from build123d import *

# Parameters (mm, degrees)
SKETCH2_R      = 7.9375
EXTRUDE1_DEPTH = 354.091885747
SKETCH3_R      = 186.436
SKETCH3_R_2    = 12.7
EXTRUDE2_DEPTH = 12.2936
SKETCH4_R      = 186.436
SKETCH4_R_2    = 12.7
EXTRUDE4_DEPTH = 26.9875
EXTRUDE5_START = -12.7
SKETCH5_R      = 186.436
EXTRUDE5_DEPTH = 12.7
EXTRUDE6_DEPTH = 351.045637854


with BuildPart() as part:
    # Sketch1 → Revolve1 (revolve)
    with BuildSketch(Plane(origin=(0, 0, 0), x_dir=(0, 0, -1), z_dir=(1, 0, 0)), mode=Mode.PRIVATE) as revolve1_sk:
        with BuildLine():
            Line((45.339, 0), (-45.339, 0))
            Line((-45.339, 0), (-45.339, 195.961))
            ThreePointArc((-45.339, 195.961), (0, 241.3), (45.339, 195.961))
            Line((45.339, 195.961), (45.339, 0))
        make_face()
    revolve(revolve1_sk.sketch.rotate(Axis((0, 0, 45.339), (0, 0, -1)), 90), axis=Axis((0, 0, 45.339), (0, 0, -1)))

    # Sketch2 → Extrude1 (cut, through all)
    with BuildSketch(Plane.XY.offset(45.339)):
        Circle(SKETCH2_R)
    extrude(amount=-EXTRUDE1_DEPTH, mode=Mode.SUBTRACT)

    # Sketch3 → Extrude2 (cut)
    with BuildSketch(Plane(origin=(0, 0, -45.339), x_dir=(-1, 0, 0), z_dir=(0, 0, -1))):
        Circle(SKETCH3_R)
        Circle(SKETCH3_R_2, mode=Mode.SUBTRACT)
    extrude(amount=-EXTRUDE2_DEPTH, mode=Mode.SUBTRACT)

    # Sketch4 → Extrude4 (cut)
    with BuildSketch(Plane(origin=(0, 0, -33.0454), x_dir=(-1, 0, 0), z_dir=(0, 0, -1))):
        Circle(SKETCH4_R)
        Circle(SKETCH4_R_2, mode=Mode.SUBTRACT)
    extrude(amount=-EXTRUDE4_DEPTH, mode=Mode.SUBTRACT)

    # Sketch5 → Extrude5 (cut)
    with BuildSketch(Plane.XY.offset(45.339).offset(EXTRUDE5_START)):
        with Locations(Location((0, 0, 0), (0, 0, 180))):
            Circle(SKETCH5_R)
    extrude(amount=EXTRUDE5_DEPTH, mode=Mode.SUBTRACT)

    # Sketch6 → Extrude6 (cut, through all)
    with BuildSketch(Plane.XY.offset(32.639)):
        with BuildLine():
            Line((150.489255243, 72.265671034), (80.015659908, 49.367411845))
            ThreePointArc((80.015659908, 49.367411845), (65.746331533, 21.36227807), (93.751465308, 7.092949695))
            Line((93.751465308, 7.092949695), (164.225060643, 29.991208884))
            ThreePointArc((164.225060643, 29.991208884), (158.770455984, 51.587648329), (150.489255243, 72.265671034))
        make_face()
        with BuildLine():
            Line((-22.225, 165.455107291), (-22.225, 91.354783989))
            ThreePointArc((-22.225, 91.354783989), (0, 69.129783989), (22.225, 91.354783989))
            Line((22.225, 91.354783989), (22.225, 165.455107291))
            ThreePointArc((22.225, 165.455107291), (0, 166.941136793), (-22.225, 165.455107291))
        make_face()
        with BuildLine():
            Line((115.232474682, -120.792466372), (71.677397455, -60.844045532))
            ThreePointArc((71.677397455, -60.844045532), (40.633467523, -55.927170065), (35.716592055, -86.971099997))
            Line((35.716592055, -86.971099997), (79.271669282, -146.919520837))
            ThreePointArc((79.271669282, -146.919520837), (98.125538208, -135.058216725), (115.232474682, -120.792466372))
        make_face()
        with BuildLine():
            Line((-79.271669282, -146.919520837), (-35.716592055, -86.971099997))
            ThreePointArc((-35.716592055, -86.971099997), (-40.633467523, -55.927170065), (-71.677397455, -60.844045532))
            Line((-71.677397455, -60.844045532), (-115.232474682, -120.792466372))
            ThreePointArc((-115.232474682, -120.792466372), (-98.125538208, -135.058216725), (-79.271669282, -146.919520837))
        make_face()
        with BuildLine():
            Line((-164.225060643, 29.991208884), (-93.751465308, 7.092949695))
            ThreePointArc((-93.751465308, 7.092949695), (-65.746331533, 21.36227807), (-80.015659908, 49.367411845))
            Line((-80.015659908, 49.367411845), (-150.489255243, 72.265671034))
            ThreePointArc((-150.489255243, 72.265671034), (-158.770455984, 51.587648329), (-164.225060643, 29.991208884))
        make_face()
    extrude(amount=-EXTRUDE6_DEPTH, mode=Mode.SUBTRACT)


solid = part.part
The listing builds one solid part. Answer for the finished solid, in the listing's coordinates (mm). A direction names the side the tool comes from. Round coordinates to 2 decimals unless told otherwise and drop trailing zeros. Write each loop counter-clockwise with the first axis right and the second up, starting at its lowest first coordinate (ties: lowest second). Pieces come first, ordered by that corner, then holes. Notation, with made-up numbers: (-16, 43) - (-6, 43) arc R24 cw to (-6, 82) - close; hole circle Ø7 at (83.25, 62). An arc over 180 degrees is marked (long way). Use a Markdown table: item, result. Add a question column.
1. The part is cut by section D-D (z = -15). Write down the section's boundary in (x, y) (1 decimal).
2. Flat-ended cylindrical pins translate along their axes: P1, Ø4, axis at y = 138, z = -16, coming from the +X side; P2, Ø8, axis at x = -144.5, z = -16.5, coming from the +Y side; P3, Ø19.5, axis at y = 138, z = 20.5, coming from the +X side. Find the tip coordinate at first contact, or state that the pin passes through.
3. Consider line 1 (Y direction, x = 0, z = 0); line 2 (Y direction, x = 0, z = -34.5); line 3 (Y direction, x = 0, z = -16.5). Determine where each line is inside the solid, lowest interval first.
4. The part is cut by section A-A (y = 0). Write down the section's boundary in (x, z), and give its area (3 significant figures).
5. A tool of negligible diameter and unlimited length cuts with its end or side. For faces 1 (the face through (22.225, 128, 14)), 2 (the face through (3, 39, 32.639)), 3 (the face through (2.75, -12.4, -25.97)), from which of +Z, -Z, +X, -X, +Y, -Y can it reach the whole face along a straight path? Write none if from no direction.
6. The part is cut by section B-B (x = 0). Write down the section's boundary in (y, z), and give its area (3 significant figures).
7. The part is cut by section C-C (z = 21). Give the number of separate pieces and of enclosed holes in the cut face, and give its area (3 significant figures).
8. For a pull along X with two mould halves and no side action, classify faces 4 (the face through (-57.799, -117.365, 13.561)), 5 (the face through (-0.2, 8.3, -45.339)) as +X half, -X half, draft (parallel to the pull), parting line (faces both ways), or undercut.
Reported:
| question | item | result |
|---|---|---|
| 1 | outline | circle Ø477.5 at (0, 0); circle Ø25.4 at (0, 0); hole circle Ø372.9 at (0, 0); hole circle Ø15.9 at (0, 0) |
| 2 | P1 | x = 196.04 |
| 2 | P2 | y = 192.85 |
| 2 | P3 | x = 200.28 |
| 3 | line 1 | -241.3 to -7.94, 7.94 to 69.13, 166.94 to 241.3 |
| 3 | line 2 | -225.38 to -186.44, -12.7 to -7.94, 7.94 to 12.7, 186.44 to 225.38 |
| 3 | line 3 | -238.19 to -186.44, -12.7 to -7.94, 7.94 to 12.7, 186.44 to 238.19 |
| 4 | outline | (-195.96, -45.34) - (-186.44, -45.34) - (-186.44, -6.06) - (-12.7, -6.06) - (-12.7, -45.34) - (-7.94, -45.34) - (-7.94, 32.64) - (-186.44, 32.64) - (-186.44, 45.34) - (-195.96, 45.34) arc R45.34 ccw to start; (7.94, -45.34) - (12.7, -45.34) - (12.7, -6.06) - (186.44, -6.06) - (186.44, -45.34) - (195.96, -45.34) arc R45.34 ccw to (195.96, 45.34) - (186.44, 45.34) - (186.44, 32.64) - (7.94, 32.64) - close |
| 4 | area | 22,400 mm^2 |
| 5 | face 1 | +Z, -Z |
| 5 | face 2 | +Z |
| 5 | face 3 | -Z |
| 6 | outline | (-195.96, -45.34) - (-186.44, -45.34) - (-186.44, -6.06) - (-12.7, -6.06) - (-12.7, -45.34) - (-7.94, -45.34) - (-7.94, 32.64) - (-186.44, 32.64) - (-186.44, 45.34) - (-195.96, 45.34) arc R45.34 ccw to start; (7.94, -45.34) - (12.7, -45.34) - (12.7, -6.06) - (69.13, -6.06) - (69.13, 32.64) - (7.94, 32.64) - close; (166.94, -6.06) - (186.44, -6.06) - (186.44, -45.34) - (195.96, -45.34) arc R45.34 ccw to (195.96, 45.34) - (186.44, 45.34) - (186.44, 32.64) - (166.94, 32.64) - close |
| 6 | area | 18,600 mm^2 |
| 7 | separate pieces | 1 |
| 7 | enclosed holes | 6 |
| 7 | area | 154,000 mm^2 |
| 8 | face 4 | undercut |
| 8 | face 5 | draft |
